```python
from build123d import *

# Parameters (mm, degrees)
F1_DEPTH = 3.175
F2_D     = 1.524


with BuildPart() as f1:
    # F0 (on Front) → F1 (new body)
    with BuildSketch(Plane.XZ):
        with BuildLine():
            Line((-3.81, 6.35), (-3.81, 0))
            Line((-3.81, 0), (-1.5875, 0))
            Line((-1.5875, 0), (-1.5875, 3.175))
            Line((-1.5875, 3.175), (1.5875, 3.175))
            Line((1.5875, 3.175), (1.5875, 0))
            Line((1.5875, 0), (3.81, 0))
            Line((3.81, 0), (3.81, 6.35))
            ThreePointArc((3.81, 6.35), (0, 10.16), (-3.81, 6.35))
        make_face()
    extrude(amount=F1_DEPTH)

    # F2 (through all)
    with Locations(Plane(origin=(0, 0, 0), x_dir=(1, 0, 0), z_dir=(0, 1, 0))):
        with Locations((0, -6.35)):
            Hole(F2_D / 2)


solid = f1.part
```
Work out the finished part from the listing and answer in its coordinate system (mm). A direction names the side the tool comes from. Give positions to 0.01 mm unless a question says otherwise; leave off trailing zeros. Loops run counter-clockwise (first coordinate to the right, second up) from the corner with the lowest first, then second, coordinate; pieces in that order, holes last. Notation, with made-up numbers: M 46,27.25 L 97,27.25 A14 cw 97,47.25 Z; hole C -14.75,5.5 d10. An arc over 180 degrees is marked long. One line per item, written item: value. Start each with the question number.
1. Determine the mould class of faces 1 (the face through (3.81, -2, 3)), 2 (the face through (3, -2, 0)), 3 (the face through (0.165, -1.61, 7.094)) for opening direction X: released by +X, released by -X, zero draft, split by the parting line, or undercut.
2. Each of these flat-tipped pins is pushed along its axis until it touches: P1, Ø1, axis at x = 0.5, y = -1.5, coming from the -Z side (3 decimals); P2, Ø1.4, axis at x = 0, z = 6.35, coming from the +Y side; P3, Ø1, axis at x = 1.5, y = -0.5, coming from the +Z side; P4, Ø1, axis at x = 2.5, y = -2, coming from the +Z side. Where does it stop, or does it pass through?
3. Find section D-D (x = -2.5). Give the vertices of the cut face in (y, z) (3 decimals).
4. Which of the six approach directions +Z, -Z, +X, -X, +Y, -Y give full straight-line access (tool end or side, diameter ignored) to faces 4 (the face through (1.588, -2, 2)), 5 (the face through (-3.81, -2, 3))?
5. Find section C-C (z = 7). Give the vertices of the cut face in (x, y) (3 decimals), and give its area (3 significant figures).
6. Find the intervals of material crossed by probe 1 along X at (y, z) = (-1.8, 6.35); probe 2 along Z at (x, y) = (0, -2.5) (3 decimals); probe 3 along X at (y, z) = (-1.3, 3), in increasing order.
7. Find section A-A (x = 0). Give the vertices of the cut face in (y, z) (3 decimals).
Reported:
1. face 1: released by +X
1. face 2: zero draft
1. face 3: undercut
2. P1: stops at z = 3.175
2. P2: passes through
2. P3: stops at z = 10.03
2. P4: stops at z = 9.59
3. outline: M -3.175,0 L 0,0 L 0,9.225 L -3.175,9.225 Z
4. face 4: -Z, +Y, -Y
4. face 5: +Z, -Z, -X, +Y, -Y
5. outline: M -3.754,-3.175 L -0.398,-3.175 L -0.398,0 L -3.754,0 Z; M 0.398,-3.175 L 3.754,-3.175 L 3.754,0 L 0.398,0 Z
5. area: 21.3 mm²
6. probe 1: x = -3.81 to -0.76, 0.76 to 3.81
6. probe 2: z = 3.175 to 5.588, 7.112 to 10.16
6. probe 3: x = -3.81 to -1.59, 1.59 to 3.81
7. outline: M -3.175,3.175 L 0,3.175 L 0,5.588 L -3.175,5.588 Z; M -3.175,7.112 L 0,7.112 L 0,10.16 L -3.175,10.16 Z
